Can you work these out from the model? Positions are in its coordinate system, mm. Give positions to 0.01 mm unless a question says otherwise; leave off trailing zeros. Loops run counter-clockwise (first coordinate to the right, second up) from the corner with the lowest first, then second, coordinate; pieces in that order, holes last. Notation, with made-up numbers: M 47,36 L 70,36 A22 cw 70,57 Z; hole C 64,26.25 d1. An arc over 180 degrees is marked long. One line per item, written item: value. Start each with the question number.
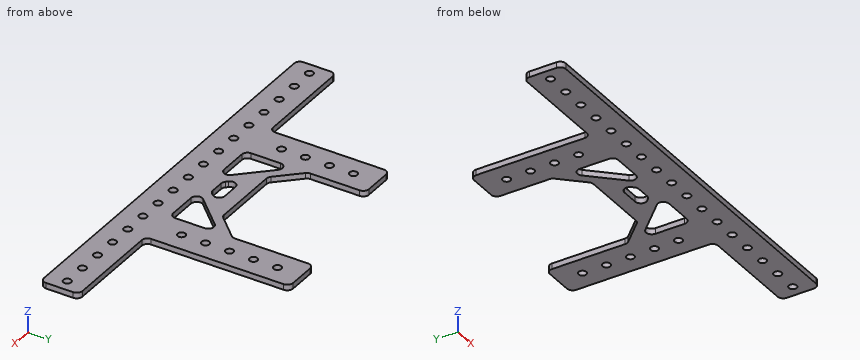
from build123d import *

# Parameters (mm, degrees)
SKETCH1_R           = 2.07
BOSS_EXTRUDE1_DEPTH = 1.5
FILLET3_R           = 3
BOSS_EXTRUDE5_DEPTH = 3
BOSS_EXTRUDE6_DEPTH = 3
FILLET4_R           = 3


with BuildPart() as part:
    # Sketch1 → Boss-Extrude1 (new, symmetric)
    with BuildSketch(Plane.XY):
        Polygon((-107.95, 10.16), (-52.07, 10.16), (-52.07, 73.66), (-31.75, 73.66), (-31.75, 10.16), (31.75, 10.16), (31.75, 86.36), (52.07, 86.36), (52.07, 10.16), (107.95, 10.16), (107.95, -10.16), (-107.95, -10.16), align=None)
        Circle(SKETCH1_R, mode=Mode.SUBTRACT)
        with Locations((12.7, 0)):
            Circle(SKETCH1_R, mode=Mode.SUBTRACT)
        with Locations((25.4, 0)):
            Circle(SKETCH1_R, mode=Mode.SUBTRACT)
        with Locations((38.1, 0)):
            Circle(SKETCH1_R, mode=Mode.SUBTRACT)
        with Locations((50.8, 0)):
            Circle(SKETCH1_R, mode=Mode.SUBTRACT)
        with Locations((63.5, 0)):
            Circle(SKETCH1_R, mode=Mode.SUBTRACT)
        with Locations((76.2, 0)):
            Circle(SKETCH1_R, mode=Mode.SUBTRACT)
        with Locations((88.9, 0)):
            Circle(SKETCH1_R, mode=Mode.SUBTRACT)
        with Locations((101.6, 0)):
            Circle(SKETCH1_R, mode=Mode.SUBTRACT)
        with Locations((-12.7, 0)):
            Circle(SKETCH1_R, mode=Mode.SUBTRACT)
        with Locations((-25.4, 0)):
            Circle(SKETCH1_R, mode=Mode.SUBTRACT)
        with Locations((-38.1, 0)):
            Circle(SKETCH1_R, mode=Mode.SUBTRACT)
        with Locations((-50.8, 0)):
            Circle(SKETCH1_R, mode=Mode.SUBTRACT)
        with Locations((-63.5, 0)):
            Circle(SKETCH1_R, mode=Mode.SUBTRACT)
        with Locations((-76.2, 0)):
            Circle(SKETCH1_R, mode=Mode.SUBTRACT)
        with Locations((-88.9, 0)):
            Circle(SKETCH1_R, mode=Mode.SUBTRACT)
        with Locations((-101.6, 0)):
            Circle(SKETCH1_R, mode=Mode.SUBTRACT)
        with Locations((-41.91, 60.96)):
            Circle(SKETCH1_R, mode=Mode.SUBTRACT)
        with Locations(Location((41.91, 60.96, 0), (0, 0, 180))):
            Circle(SKETCH1_R, mode=Mode.SUBTRACT)
        with Locations((-41.91, 48.26)):
            Circle(SKETCH1_R, mode=Mode.SUBTRACT)
        with Locations(Location((41.91, 48.26, 0), (0, 0, 180))):
            Circle(SKETCH1_R, mode=Mode.SUBTRACT)
        with Locations((-41.91, 35.56)):
            Circle(SKETCH1_R, mode=Mode.SUBTRACT)
        with Locations(Location((41.91, 35.56, 0), (0, 0, 180))):
            Circle(SKETCH1_R, mode=Mode.SUBTRACT)
        with Locations((-41.91, 22.86)):
            Circle(SKETCH1_R, mode=Mode.SUBTRACT)
        with Locations(Location((41.91, 22.86, 0), (0, 0, 180))):
            Circle(SKETCH1_R, mode=Mode.SUBTRACT)
        with Locations((41.91, 73.66)):
            Circle(SKETCH1_R, mode=Mode.SUBTRACT)
    extrude(amount=BOSS_EXTRUDE1_DEPTH, both=True)

    # Fillet3
    fillet3_edges = [part.edges().sort_by_distance(p)[0] for p in [
        (107.95, -10.16, 0),
        (-107.95, -10.16, 0),
        (-107.95, 10.16, 0),
        (-52.07, 10.16, 0),
        (-52.07, 73.66, 0),
        (-31.75, 10.16, 0),
        (31.75, 10.16, 0),
        (52.07, 86.36, 0),
        (52.07, 10.16, 0),
        (107.95, 10.16, 0),
    ]]
    fillet(fillet3_edges, radius=FILLET3_R)

    # Sketch3 → Boss-Extrude5 (add)
    with BuildSketch(Plane.XY.offset(1.5)):
        Polygon((-4.77443609, 15.16), (-31.75, 43.41), (-31.75, 36.169972042), (-6.913410156, 10.16), (6.913410156, 10.16), (31.75, 36.169972042), (31.75, 43.41), (4.77443609, 15.16), align=None)
    extrude(amount=-BOSS_EXTRUDE5_DEPTH)

    # Sketch4 → Boss-Extrude6 (add)
    with BuildSketch(Plane.XY.offset(1.5)):
        Polygon((19.097744361, 30.16), (-19.097744361, 30.16), (-11.458646617, 22.16), (11.458646617, 22.16), align=None)
    extrude(amount=-BOSS_EXTRUDE6_DEPTH)

    # Fillet4
    fillet4_edges = [part.edges().sort_by_distance(p)[0] for p in [
        (-31.75, 73.66, 0),
        (-31.75, 36.169972042, 0),
        (31.75, 86.36, 0),
        (-31.75, 43.41, 0),
        (-4.77443609, 15.16, 0),
        (4.77443609, 15.16, 0),
        (31.75, 43.41, 0),
        (31.75, 36.169972042, 0),
        (6.913410156, 10.16, 0),
        (-6.913410156, 10.16, 0),
        (19.097744361, 30.16, 0),
        (11.458646617, 22.16, 0),
        (-11.458646617, 22.16, 0),
        (-19.097744361, 30.16, 0),
    ]]
    fillet(fillet4_edges, radius=FILLET4_R)


solid = part.part
Q1. For P1, Ø1.5, axis at y = 59, z = 0, coming from the -X side; P2, Ø3.5, axis at x = 41.91, y = 60.96, coming from the -Z side, each with a flat end and sliding along its axis, tell me the tip position at first contact or that it passes through.
Q2. If we section it at B-B, the plane x = 0: Write out the boundary of the cut face in (y, z).
Q3. If we section it at A-A, the plane x = -76.2: Write out the boundary of the cut face in (y, z).
Q4. I need wall thicknesses on line 1 along Y through (x, z) = (41.91, -0.75); line 2 along Y through (x, z) = (-89, 0.1); line 3 along X through (y, z) = (20, -0.5). Which ranges of each line are inside material? Lowest first, please.
Q5. If we section it at C-C, the plane y = 0: Give the number of separate pieces and of enclosed holes in the cut face, plus the area to 3 significant figures.
Response:
1. P1: x = -52.07
1. P2: through
2. outline: M -10.16,-1.5 L -2.07,-1.5 L -2.07,1.5 L -10.16,1.5 Z; M 2.07,-1.5 L 15.16,-1.5 L 15.16,1.5 L 2.07,1.5 Z; M 22.16,-1.5 L 30.16,-1.5 L 30.16,1.5 L 22.16,1.5 Z
3. outline: M -10.16,-1.5 L -2.07,-1.5 L -2.07,1.5 L -10.16,1.5 Z; M 2.07,-1.5 L 10.16,-1.5 L 10.16,1.5 L 2.07,1.5 Z
4. line 1: -10.16 to 20.79, 24.93 to 33.49, 37.63 to 46.19, 50.33 to 58.89, 63.03 to 71.59, 75.73 to 86.36
4. line 2: -10.16 to -2.07, 2.07 to 10.16
4. line 3: -52.07 to -31.75, -16.31 to -7.33, 7.33 to 16.31, 31.75 to 52.07
5. separate pieces: 18
5. enclosed holes: 0
5. area: 437 mm^2
